Geometry check sheet. Reference: the model listing, model coordinates, mm. A direction names the side the tool comes from. Coordinates: 2 decimals unless noted, no trailing zeros. Write each loop counter-clockwise with the first axis right and the second up, starting at its lowest first coordinate (ties: lowest second). Pieces come first, ordered by that corner, then holes.
from build123d import *

# Parameters (mm, degrees)
SKETCH1_R               = 3.25
BOSS_EXTRUDE1_DEPTH     = 40
BOSS_EXTRUDE2_START     = -30
SKETCH10_R              = 3.25
BOSS_EXTRUDE2_DEPTH     = 30
SKETCH2_R               = 3
SKETCH2_R_2             = 5
CUT_EXTRUDE1_DEPTH      = 10.669417382
SKETCH8_R               = 1.6
SKETCH8_R_2             = 2.6
CUT_EXTRUDE2_DEPTH      = 45.768898873
SKETCH11_R              = 3.25
BOSS_EXTRUDE3_DEPTH     = 10
CUT_EXTRUDE3_DEPTH      = 48.949888605
CUT_EXTRUDE3_DEPTH_BACK = 48.949888605
SKETCH12_R              = 3.25
SKETCH13_R              = 3.25
BOSS_EXTRUDE4_DEPTH     = 2


with BuildPart() as part:
    # Sketch1 → Boss-Extrude1 (new body)
    with BuildSketch(Plane.XY):
        with BuildLine():
            Line((-11.919417382, 0), (11.919417382, 0))
            Line((11.919417382, 0), (11.919417382, 4))
            ThreePointArc((11.919417382, 4), (13.274247078, 10.811188835), (7.5, 14.669417382))
            Line((7.5, 14.669417382), (-7.5, 14.669417382))
            ThreePointArc((-7.5, 14.669417382), (-13.274247078, 10.811188835), (-11.919417382, 4))
            Line((-11.919417382, 4), (-11.919417382, 0))
        make_face()
        with Locations((7.5, 8.419417382)):
            Circle(SKETCH1_R, mode=Mode.SUBTRACT)
        with Locations((-7.5, 8.419417382)):
            Circle(SKETCH1_R, mode=Mode.SUBTRACT)
    extrude(amount=BOSS_EXTRUDE1_DEPTH)

    # Sketch10 → Boss-Extrude2 (add)
    with BuildSketch(Plane.XY.offset(40).offset(BOSS_EXTRUDE2_START)):
        with Locations((7.5, 8.419417382)):
            Circle(SKETCH10_R)
        with Locations((-7.5, 8.419417382)):
            Circle(SKETCH10_R)
    extrude(amount=BOSS_EXTRUDE2_DEPTH)

    # Sketch2 → Cut-Extrude1 (cut)
    with BuildSketch(Plane(origin=(0, 14.669417382, 0), x_dir=(1, 0, 0), z_dir=(0, 1, 0))):
        with Locations((0, -7.5)):
            Circle(SKETCH2_R)
        with Locations((0, -11.5)):
            Circle(SKETCH2_R)
        with Locations(Location((0, -32, 0), (0, 0, 180))):
            Circle(SKETCH2_R_2)
    extrude(amount=-CUT_EXTRUDE1_DEPTH, mode=Mode.SUBTRACT)

    # Sketch8 → Cut-Extrude2 (cut, through all)
    with BuildSketch(Plane(origin=(0, 14.669417382, 0), x_dir=(1, 0, 0), z_dir=(0, 1, 0))):
        with Locations(Location((0, -7.5, 0), (0, 0, 180))):
            Circle(SKETCH8_R)
        with Locations(Location((0, -11.5, 0), (0, 0, 180))):
            Circle(SKETCH8_R)
        with Locations(Location((0, -32, 0), (0, 0, 180))):
            Circle(SKETCH8_R_2)
    extrude(amount=-CUT_EXTRUDE2_DEPTH, mode=Mode.SUBTRACT)

    # Sketch11 → Boss-Extrude3 (add)
    # profile 1 of 2: a face of its own
    with BuildSketch(Plane.XZ):
        with BuildLine():
            Line((-15.75, 27.5), (-11.919417382, 27.5))
            Line((-11.919417382, 27.5), (-11.919417382, 40))
            Line((-11.919417382, 40), (-15.75, 40))
            ThreePointArc((-15.75, 40), (-22, 33.75), (-15.75, 27.5))
        make_face()
        with Locations(Location((-15.75, 33.75, 0), (0, 0, 270))):
            Circle(SKETCH11_R, mode=Mode.SUBTRACT)
    # profile 2 of 2: a face of its own
    with BuildSketch(Plane.XZ):
        with BuildLine():
            Line((15.75, 40), (11.919417382, 40))
            Line((11.919417382, 40), (11.919417382, 27.5))
            Line((11.919417382, 27.5), (15.75, 27.5))
            ThreePointArc((15.75, 27.5), (22, 33.75), (15.75, 40))
        make_face()
        with Locations(Location((15.75, 33.75, 0), (0, 0, 270))):
            Circle(SKETCH11_R, mode=Mode.SUBTRACT)
    extrude(amount=-BOSS_EXTRUDE3_DEPTH)

    # Sketch12 → Cut-Extrude3 (cut, two sides: drawn at the far end of the back side and taken through both)
    with BuildSketch(Plane.XZ.offset(-CUT_EXTRUDE3_DEPTH_BACK)):
        with Locations(Location((15.75, 33.75, 0), (0, 0, 270))):
            Circle(SKETCH12_R)
        with Locations(Location((-15.75, 33.75, 0), (0, 0, 270))):
            Circle(SKETCH12_R)
    extrude(amount=CUT_EXTRUDE3_DEPTH + CUT_EXTRUDE3_DEPTH_BACK, mode=Mode.SUBTRACT)

    # Sketch13 → Boss-Extrude4 (add)
    with BuildSketch(Plane.XZ):
        with Locations(Location((15.75, 33.75, 0), (0, 0, 270))):
            Circle(SKETCH13_R)
        with Locations(Location((-15.75, 33.75, 0), (0, 0, 270))):
            Circle(SKETCH13_R)
    extrude(amount=-BOSS_EXTRUDE4_DEPTH)


solid = part.part
1. Access from +Z, -Z, +X, -X, +Y, -Y to the whole of each face (thin tool, end or side, straight path). Record for faces 4 (the flat face through (-2, 4, 30)), 5 (the flat face through (19, 10, 35)), 6 (the cylindrical face through (-10.08, 6.44, 4.93)), 7 (the cylindrical face through (-22, 4.9, 33.9)), 8 (the flat face through (-19, 10, 32)).
Computed values:
face 4: +Y
face 5: +Z, -Z, +X, +Y
face 6: -Z
face 7: -X, +Y, -Y
face 8: +Z, -Z, -X, +Y
2. Sectioned sample at B-B, the plane x = 0. Record the boundary of the cut face in (y, z).
Computed values:
outline: (0, 0) - (14.67, 0) - (14.67, 4.5) - (4, 4.5) - (4, 5.9) - (0, 5.9) - close; (0, 9.1) - (4, 9.1) - (4, 9.9) - (0, 9.9) - close; (0, 13.1) - (4, 13.1) - (4, 14.5) - (14.67, 14.5) - (14.67, 27) - (4, 27) - (4, 29.4) - (0, 29.4) - close; (0, 34.6) - (4, 34.6) - (4, 37) - (14.67, 37) - (14.67, 40) - (0, 40) - close
3. Sectioned sample at D-D, the plane y = 10.5. Record the boundary of the cut face in (x, z), and give its area (3 significant figures).
Computed values:
outline: (-13.39, 0) - (-10, 0) - (-10, 10) - (-5, 10) - (-5, 0) - (5, 0) - (5, 10) - (10, 10) - (10, 0) - (13.39, 0) - (13.39, 31.51) arc R3.25 cw to (13.39, 35.99) - (13.39, 40) - (-13.39, 40) - (-13.39, 35.99) arc R3.25 cw to (-13.39, 31.51) - close; hole circle Ø10 at (0, 32); hole (-2.24, 9.5) arc R3 ccw (long way) to (2.24, 9.5) arc R3 ccw (long way) to start
area: 837 mm2
4. Sectioned sample at A-A, the plane y = 1.5. Record the boundary of the cut face in (x, z), and give its area (3 significant figures).
Computed values:
outline: (-15.75, 27.5) - (-11.92, 27.5) - (-11.92, 0) - (11.92, 0) - (11.92, 27.5) - (15.75, 27.5) arc R6.25 ccw to (15.75, 40) - (-15.75, 40) arc R6.25 ccw to start; hole circle Ø5.2 at (0, 32); hole circle Ø3.2 at (0, 7.5); hole circle Ø3.2 at (0, 11.5)
area: 1,130 mm2
5. Thickness scan on line 1 along Z through (x, y) = (0, 10.25); line 2 along X through (y, z) = (6, 33.75); line 3 along X through (y, z) = (2.5, 33.5) (3 decimals). Record the ranges inside material, lowest first.
Computed values:
line 1: z = 0 to 4.5, 14.5 to 27, 37 to 40
line 2: x = -22 to -19, -12.5 to -4.68, 4.68 to 12.5, 19 to 22
line 3: x = -21.995 to -18.99, -12.51 to -2.124, 2.124 to 12.51, 18.99 to 21.995
6. Sectioned sample at C-C, the plane z = 11.5. Record the boundary of the cut face in (x, y).
Computed values:
outline: (-11.92, 0) - (-1.6, 0) - (-1.6, 4) - (-3, 4) - (-3, 14.67) - (-7.5, 14.67) arc R6.25 ccw to (-11.92, 4) - close; (1.6, 0) - (11.92, 0) - (11.92, 4) arc R6.25 ccw to (7.5, 14.67) - (3, 14.67) - (3, 4) - (1.6, 4) - close
7. Gauge pin test, flat ends, axial feed: pin 1 Ø6 at (x, z) = (15.75, 33.75) entering from +Y; pin 2 Ø8.5 at (x, z) = (0, 32) entering from +Y; pin 3 Ø3 at (x, z) = (0, 7.5) entering from -Y; pin 4 Ø6 at (y, z) = (8, 9.5) entering from -X. Record the tip position at first contact, or that the pin passes through.
Computed values:
pin 1: stops at y = 2
pin 2: stops at y = 4
pin 3: passes through
pin 4: stops at x = -13.75
8. Draft check along Y on faces 1 (the cylindrical face through (0.338, 2.028, 34.578)), 2 (the flat face through (-8, 8, 10)), 3 (the cylindrical face through (13.31, 10.72, 15.28)). Enter one of: released by +Y, released by -Y, zero draft, split by the parting line, or undercut.
Computed values:
face 1: zero draft
face 2: undercut
face 3: split by the parting line
